Here's how the part is built. I have some questions about the finished solid (model axes, mm). Coordinates: 2 decimals unless noted, no trailing zeros. Order: outer loops, then holes, each group sorted by start corner. A loop starts at its lowest first (then second) coordinate and runs counter-clockwise, first axis right, second up. Notation, with made-up numbers: (-0.75, -2) - (49.25, -2) arc R26 ccw to (49.25, 19) - close; hole circle Ø10 at (53, 21). An arc over 180 degrees is marked (long way). Use CSV: the item, a comma, the result in double quotes. Start each with the question number.
from build123d import *

# Parameters (mm, degrees)
BOSS_EXTRUDE1_DEPTH       = 20
SKETCH2_W                 = 20
SKETCH2_H                 = 20
BOSS_EXTRUDE2_DEPTH       = 250
DRAFT5_ANGLE              = 5
FILLET1_R                 = 5
DRAFT5_OF_MIRROR2_2_ANGLE = 5
FILLET1_OF_MIRROR2_R      = 5


with BuildPart() as part:
    # Sketch1 → Boss-Extrude1 (new body)
    with BuildSketch(Plane(origin=(0, 0, 0), x_dir=(0, 0, -1), z_dir=(1, 0, 0))):
        with BuildLine():
            Line((-824.175, -50), (824.175, -50))
            ThreePointArc((824.175, -50), (901.175, 27), (824.175, 104))
            Line((824.175, 104), (-824.175, 104))
            ThreePointArc((-824.175, 104), (-901.175, 27), (-824.175, -50))
        make_face()
    extrude(amount=BOSS_EXTRUDE1_DEPTH)

    # Sketch2 → Boss-Extrude2 (add)
    with BuildSketch(Plane.XZ.offset(50)):
        with Locations((10, 814.175)):
            Rectangle(SKETCH2_W, SKETCH2_H)
    boss_extrude2 = extrude(amount=BOSS_EXTRUDE2_DEPTH)

    # Draft5
    draft5_faces = [part.faces().sort_by_distance(p)[0] for p in [
        (10, -175, 824.175),
        (10, -175, 804.175),
    ]]
    draft(draft5_faces, Plane(origin=(0, -300, 0), x_dir=(0, 0, -1), z_dir=(0, -1, 0)), DRAFT5_ANGLE)

    # Fillet1
    fillet1_edges = [part.edges().sort_by_distance(p)[0] for p in [
        (0, -173.371611905, 835.253548439),
        (0, -175, 793.238917059),
        (20, -175, 793.238917059),
        (20, -173.371611905, 835.253548439),
    ]]
    fillet(fillet1_edges, radius=FILLET1_R)

    # Mirror2: Boss-Extrude2 across plane
    add(boss_extrude2.mirror(Plane.XY))

    # Draft5 of Mirror2 2
    draft5_of_mirror2_2_faces = [part.faces().sort_by_distance(p)[0] for p in [
        (10, -175, -824.175),
        (10, -175, -804.175),
    ]]
    draft(draft5_of_mirror2_2_faces, Plane(origin=(0, -300, 0), x_dir=(0, 0, 1), z_dir=(0, -1, 0)), DRAFT5_OF_MIRROR2_2_ANGLE)

    # Fillet1 of Mirror2
    fillet1_of_mirror2_edges = [part.edges().sort_by_distance(p)[0] for p in [
        (0, -173.371611905, -835.253548439),
        (0, -175, -793.238917059),
        (20, -175, -793.238917059),
        (20, -173.371611905, -835.253548439),
    ]]
    fillet(fillet1_of_mirror2_edges, radius=FILLET1_OF_MIRROR2_R)


solid = part.part
Item 1: For pin 1 Ø3 at (x, z) = (13, 462) entering from -Y; pin 2 Ø4 at (x, y) = (9.5, -223.5) entering from +Z; pin 3 Ø10 at (x, y) = (9.5, 28.5) entering from -Z (3 decimals), each with a flat end and sliding along its axis, tell me the tip position at first contact or that it passes through.
Item 2: Suppose I cut it at B-B on z = 360.5. Write out the boundary of the cut face in (x, y), then the cut area to 3 significant figures.
Item 3: Suppose I cut it at A-A on x = 8.25. Write out the boundary of the cut face in (y, z) (3 decimals).
Item 4: Please list where these lines run through material, in increasing order: line 1 along Z through (x, y) = (3.5, 26.5); line 2 along Y through (x, z) = (1.5, 249); line 3 along Z through (x, y) = (7.5, -201.5). Write a range as from..to.
Here are the results:
1,pin 1,"y = -50"
1,pin 2,"z = 831.04"
1,pin 3,"z = -901.175"
2,outline,"(0, -50) - (20, -50) - (20, 104) - (0, 104) - close"
2,area,"3,080 mm^2"
3,outline,"(-300, -824.175) - (-46.743, -846.332) arc R77 ccw to (104, -824.175) - (104, 824.175) arc R77 ccw to (-46.743, 846.332) - (-300, 824.175) - (-300, 804.175) - (-50, 782.303) - (-50, -782.303) - (-300, -804.175) - close"
4,line 1,"-901.17..901.17"
4,line 2,"-50..104"
4,line 3,"-832.79..-795.56, 795.56..832.79"
